Work out the finished part from the listing and answer in its coordinate system (mm). Give positions to 0.01 mm unless a question says otherwise; leave off trailing zeros. Loops run counter-clockwise (first coordinate to the right, second up) from the corner with the lowest first, then second, coordinate; pieces in that order, holes last. Notation, with made-up numbers: (20, -32) - (63, -32) arc R18 cw to (63, -18) - close; hole circle Ø9 at (76, 8.25). An arc over 180 degrees is marked (long way). One line per question, with ' | ' between items. Start each with the question number.
1. Find the intervals of material crossed by line 1 (X direction, y = 1.35, z = -55), in increasing order.
2. For a pull along X with two mould halves and no side action, classify faces 1 (the face through (114.764, 2.958, -55.751)), 2 (the face through (-2, 0, -1)), 3 (the face through (125, 3, 1)), 4 (the face through (-110.2, 3, -55.8)) as released by +X, released by -X, zero draft, split by the parting line, or undercut.
3. This flat-tipped pin is pushed along its axis until it touches: pin 1 (3 mm diameter, centred on x = 112.38, z = -55, fed in from -Y). Where does it stop, or does it pass through?
4. Section A-A (z = 55) is taken. Determine the outline of the cut face in (x, y), plus the area to 3 significant figures.
from build123d import *

# Parameters (mm, degrees)
SKETCH1_W           = 250
SKETCH1_H           = 130
BOSS_EXTRUDE1_DEPTH = 6
SKETCH1_4_R         = 2.5
CUT_EXTRUDE1_DEPTH  = 6


with BuildPart() as part:
    # Sketch1 → Boss-Extrude1 (new body)
    with BuildSketch(Plane(origin=(0, 0, 0), x_dir=(1, 0, 0), z_dir=(0, 1, 0))):
        Rectangle(SKETCH1_W, SKETCH1_H)
    extrude(amount=BOSS_EXTRUDE1_DEPTH)

    # Sketch1<4> → Cut-Extrude1 (cut)
    with BuildSketch(Plane(origin=(0, 0, 0), x_dir=(1, 0, 0), z_dir=(0, 1, 0))):
        with Locations((-112.568736162, 55)):
            Circle(SKETCH1_4_R)
        with Locations((112.379080965, 55)):
            Circle(SKETCH1_4_R)
        with Locations((112.379080965, -55)):
            Circle(SKETCH1_4_R)
        with Locations((-112.568736162, -55)):
            Circle(SKETCH1_4_R)
    extrude(amount=CUT_EXTRUDE1_DEPTH, mode=Mode.SUBTRACT)


solid = part.part
Conclusion:
1) line 1: -125 to -115.07, -110.07 to 109.88, 114.88 to 125
2) face 1: undercut | face 2: zero draft | face 3: released by +X | face 4: undercut
3) pin 1: through
4) outline: (-125, 0) - (-115.07, 0) - (-115.07, 6) - (-125, 6) - close; (-110.07, 0) - (109.88, 0) - (109.88, 6) - (-110.07, 6) - close; (114.88, 0) - (125, 0) - (125, 6) - (114.88, 6) - close | area: 1,440 mm²
